from build123d import *

# Parameters (mm, degrees)
SKETCH2_R          = 2.54
CUT_EXTRUDE1_DEPTH = 44.818496962
SKETCH3_R          = 9.525
CUT_EXTRUDE2_DEPTH = 3.81


with BuildPart() as part:
    # Sketch1 → Revolve1 (revolve)
    with BuildSketch(Plane.XY):
        Polygon((-7.874, 8.255), (-7.874, 30.205033861), (0, 30.48), (0, 4.826), (-9.652, 4.826), (-9.652, 8.255), align=None)
    revolve(axis=Axis((0, 0, 0), (-1, 0, 0)))

    # Sketch2 → Cut-Extrude1 (cut, through all)
    with BuildSketch(Plane.ZY.offset(7.874)):
        with Locations(Location((-17.960512242, 17.960512242, 0), (0, 0, 270))):
            Circle(SKETCH2_R)
        with Locations(Location((17.960512242, 17.960512242, 0), (0, 0, 270))):
            Circle(SKETCH2_R)
        with Locations(Location((17.960512242, -17.960512242, 0), (0, 0, 270))):
            Circle(SKETCH2_R)
        with Locations(Location((-17.960512242, -17.960512242, 0), (0, 0, 270))):
            Circle(SKETCH2_R)
    extrude(amount=-CUT_EXTRUDE1_DEPTH, mode=Mode.SUBTRACT)

    # Sketch3 → Cut-Extrude2 (cut)
    with BuildSketch(Plane(origin=(0, 0, 0), x_dir=(0, 0, -1), z_dir=(1, 0, 0))):
        with Locations(Location((0, 0, 0), (0, 0, 90))):
            Circle(SKETCH3_R)
    extrude(amount=-CUT_EXTRUDE2_DEPTH, mode=Mode.SUBTRACT)


solid = part.part
Input: part model. Units: mm. Frame: model coordinates. A direction names the side the tool comes from. Round coordinates to 2 decimals unless told otherwise and drop trailing zeros. Loops run counter-clockwise (first coordinate to the right, second up) from the corner with the lowest first, then second, coordinate; pieces in that order, holes last. Notation, with made-up numbers: (-37.75, -23) -> (18.25, -23) arc R21 ccw to (18.25, -5) -> close; hole circle Ø3 at (1, 63.25). An arc over 180 degrees is marked (long way). Answer as a JSON object with one key per item and string values. Group by question number.
1) Section query C-C on x = -5. Output: boundary loops of the cut face in (y, z).
2) Section query D-D on y = 17. State how many separate pieces and enclosed holes the cut face has, plus the area to 3 significant figures.
3) Draft query along Z for faces 4 (the conical face through (-4.757, -24.056, 18.446)), 5 (the cylindrical face through (-6.772, -3.83, 2.937)), 6 (the flat face through (-7.874, -6, 6)), 7 (the cylindrical face through (-1.878, -7.559, -5.796)). Return one class per face: +Z half, -Z half, draft (parallel to the pull), parting line (faces both ways), or undercut.
4) Ray query, L1, parallel to X at y = 21.5, z = 3; L2, parallel to Z at x = -7, y = 16.5; L3, parallel to Z at x = -3.25, y = -6.5. Return the intervals inside material, ascending.
5) Section query A-A on z = 0. Output: boundary loops of the cut face in (x, y) (3 decimals).
6) Reachability of faces 1 (the flat face through (-3.81, 4, -4)), 2 (the cylindrical face through (-8.751, 7.874, -2.48)), 3 (the cylindrical face through (-3.99, 19.83, 19.68)) from +Z, -Z, +X, -X, +Y, -Y: full face, straight path, thin tool, end or side. Return the list, or none.
7) Pin query (flat end, axial travel): pin 1 (1.5 mm diameter, centred on y = -5, z = 23, fed in from -X); pin 2 (1 mm diameter, centred on x = -7, y = -13.5, fed in from -Z); pin 3 (3 mm diameter, centred on y = -17.96, z = 17.96, fed in from -X); pin 4 (2 mm diameter, centred on x = -6, z = 23.5, fed in from -Y). Return the tip coordinate at first contact, or that it passes through.
Reply:
{
 "1": {"outline": "circle Ø60.61 at (0, 0); hole circle Ø5.08 at (-17.96, -17.96); hole circle Ø5.08 at (-17.96, 17.96); hole circle Ø9.65 at (0, 0); hole circle Ø5.08 at (17.96, -17.96); hole circle Ø5.08 at (17.96, 17.96)"},
 "2": {"separate pieces": "3", "enclosed holes": "0", "area": "322 mm2"},
 "3": {"face 4": "parting line", "face 5": "undercut", "face 6": "draft", "face 7": "undercut"},
 "4": {"L1": "x = -7.87 to 0", "L2": "z = -25.34 to -20.04, -15.88 to 15.88, 20.04 to 25.34", "L3": "z = -29.66 to -6.96, 6.96 to 29.66"},
 "5": {"outline": "(-9.652, -8.255) -> (-7.874, -8.255) -> (-7.874, -30.205) -> (0, -30.48) -> (0, -9.525) -> (-3.81, -9.525) -> (-3.81, -4.826) -> (-9.652, -4.826) -> close; (-9.652, 4.826) -> (-3.81, 4.826) -> (-3.81, 9.525) -> (0, 9.525) -> (0, 30.48) -> (-7.874, 30.205) -> (-7.874, 8.255) -> (-9.652, 8.255) -> close"},
 "6": {"face 1": "+X", "face 2": "-X", "face 3": "+X, -X"},
 "7": {"pin 1": "stops at x = -7.87", "pin 2": "stops at z = -27.3", "pin 3": "passes through", "pin 4": "stops at y = -20.25"}
}
